```python
from build123d import *

# Parameters (mm, degrees)
SKETCH1_W           = 369
SKETCH1_H           = 81
BOSS_EXTRUDE1_DEPTH = 10
SKETCH2_W           = 23
SKETCH2_H           = 162
BOSS_EXTRUDE2_DEPTH = 38
SKETCH3_R           = 2.5
CUT_EXTRUDE1_DEPTH  = 163
SKETCH4_R           = 1.65
CUT_EXTRUDE2_DEPTH  = 24
CUT_EXTRUDE4_DEPTH  = 13
SKETCH6_R           = 3.3
SKETCH6_R_2         = 3.25
CUT_EXTRUDE5_DEPTH  = 13


with BuildPart() as part:
    # Sketch1 → Boss-Extrude1 (new body)
    with BuildSketch(Plane.XY):
        with Locations((184.5, 40.5)):
            Rectangle(SKETCH1_W, SKETCH1_H)
    extrude(amount=BOSS_EXTRUDE1_DEPTH)

    # Sketch2 → Boss-Extrude2 (add)
    with BuildSketch(Plane(origin=(369, 0, 0), x_dir=(0, 0, -1), z_dir=(1, 0, 0))):
        with Locations((1.5, 0)):
            Rectangle(SKETCH2_W, SKETCH2_H)
    extrude(amount=BOSS_EXTRUDE2_DEPTH)

    # Sketch3 → Cut-Extrude1 (cut, through all)
    with BuildSketch(Plane(origin=(0, 81, 0), x_dir=(1, 0, 0), z_dir=(0, 1, 0))):
        with Locations((388, 1.5)):
            Circle(SKETCH3_R)
    extrude(amount=-CUT_EXTRUDE1_DEPTH, mode=Mode.SUBTRACT)

    # Sketch4 → Cut-Extrude2 (cut, through all)
    with BuildSketch(Plane.XY.offset(10)):
        with Locations((398, -78)):
            Circle(SKETCH4_R)
        with Locations((398, 78)):
            Circle(SKETCH4_R)
    extrude(amount=-CUT_EXTRUDE2_DEPTH, mode=Mode.SUBTRACT)

    # Sketch5 → Cut-Extrude4 (cut)
    with BuildSketch(Plane.XY.offset(10)):
        with BuildLine():
            Line((394, 78), (394, 81))
            Line((394, 81), (402, 81))
            Line((402, 81), (402, 78))
            ThreePointArc((402, 78), (398, 74), (394, 78))
        make_face()
        with BuildLine():
            Line((394, -78), (394, -81))
            Line((394, -81), (402, -81))
            Line((402, -81), (402, -78))
            ThreePointArc((402, -78), (398, -74), (394, -78))
        make_face()
    extrude(amount=-CUT_EXTRUDE4_DEPTH, mode=Mode.SUBTRACT)

    # Sketch6 → Cut-Extrude5 (cut)
    with BuildSketch(Plane.XY.offset(10)):
        with Locations((10, 71)):
            Circle(SKETCH6_R)
        with Locations((40, 71)):
            Circle(SKETCH6_R)
        with Locations((40, 10)):
            Circle(SKETCH6_R)
        with Locations((10, 10)):
            Circle(SKETCH6_R_2)
    extrude(amount=-CUT_EXTRUDE5_DEPTH, mode=Mode.SUBTRACT)


solid = part.part
```
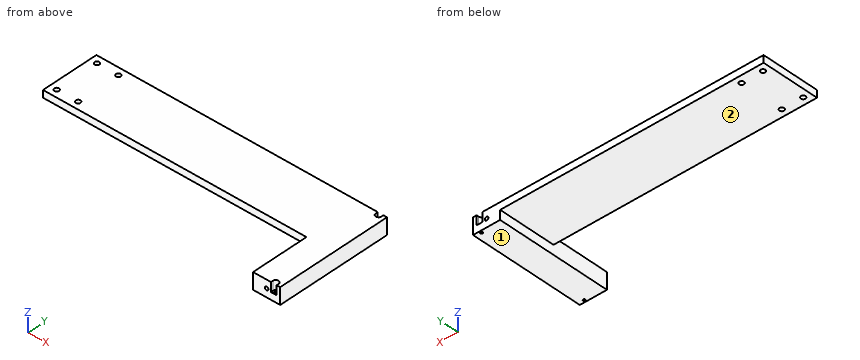
For this review, take the finished solid that the model builds, in its own axes (mm). Face numbers are marked on the shaded views. A direction names the side the tool comes from. Round coordinates to 2 decimals unless told otherwise and drop trailing zeros. Order: outer loops, then holes, each group sorted by start corner. A loop starts at its lowest first (then second) coordinate and runs counter-clockwise, first axis right, second up. Notation, with made-up numbers: (-22, 12) -> (-11, 12) arc R19 cw to (-11, 19) -> close; hole circle Ø9 at (-21, -16). An arc over 180 degrees is marked (long way). Use a Markdown table: item, result.
Item 1: For line 1 along Y through (x, z) = (10, 7); line 2 along X through (y, z) = (-78, -8.75); line 3 along Y through (x, z) = (40, 4), list the stretches that pass through material, from the lowest coordinate up. Write a range as [from, to].
Resolved:
| item | result |
|---|---|
| line 1 | y = [0, 6.75], [13.25, 67.7], [74.3, 81] |
| line 2 | x = [369, 396.35], [399.65, 407] |
| line 3 | y = [0, 6.7], [13.3, 67.7], [74.3, 81] |
Item 2: Take a section at C-C (x = 337). State the section outline as (y, z) points.
Resolved:
| item | result |
|---|---|
| outline | (0, 0) -> (81, 0) -> (81, 10) -> (0, 10) -> close |
Item 3: Take a section at D-D (y = -16). State the section outline as (x, z) points, plus the area to 3 significant figures.
Resolved:
| item | result |
|---|---|
| outline | (369, -13) -> (407, -13) -> (407, 10) -> (369, 10) -> close; hole circle Ø5 at (388, -1.5) |
| area | 854 mm² |
Item 4: Take a section at B-B (y = 41). State the section outline as (x, z) points.
Resolved:
| item | result |
|---|---|
| outline | (0, 0) -> (369, 0) -> (369, -13) -> (407, -13) -> (407, 10) -> (0, 10) -> close; hole circle Ø5 at (388, -1.5) |
Item 5: Machinability: for the marked faces 1 and 2, which of the approach directions +Z, -Z, +X, -X, +Y, -Y give a long, thin tool a straight path to every point of the face, cutting with its end or side? Answer none if there is none.
Resolved:
| item | result |
|---|---|
| face 1 | -Z, +X, -X, +Y, -Y |
| face 2 | -Z, -X, +Y, -Y |
Item 6: Take a section at A-A (z = 5.5). State the section outline as (x, y) points, plus the area to 3 significant figures.
Resolved:
| item | result |
|---|---|
| outline | (0, 0) -> (369, 0) -> (369, -81) -> (394, -81) -> (394, -78) arc R4 cw to (402, -78) -> (402, -81) -> (407, -81) -> (407, 81) -> (402, 81) -> (402, 78) arc R4 cw to (394, 78) -> (394, 81) -> (0, 81) -> close; hole circle Ø6.6 at (10, 71); hole circle Ø6.5 at (10, 10); hole circle Ø6.6 at (40, 10); hole circle Ø6.6 at (40, 71) |
| area | 35,800 mm² |
Item 7: For pin 1 (5 mm diameter, centred on y = 6.5, z = -5.5, fed in from -X); pin 2 (3 mm diameter, centred on x = 235.5, z = 5.5, fed in from -Y); pin 3 (5.5 mm diameter, centred on x = 397, y = 76.5, fed in from +Z); pin 4 (7.5 mm diameter, centred on x = 10, y = 10, fed in from -Z), all flat-tipped, find the tip position at first contact; note any pin that passes through.
Resolved:
| item | result |
|---|---|
| pin 1 | stops at x = 369 |
| pin 2 | stops at y = 0 |
| pin 3 | stops at z = 10 |
| pin 4 | stops at z = 0 |
